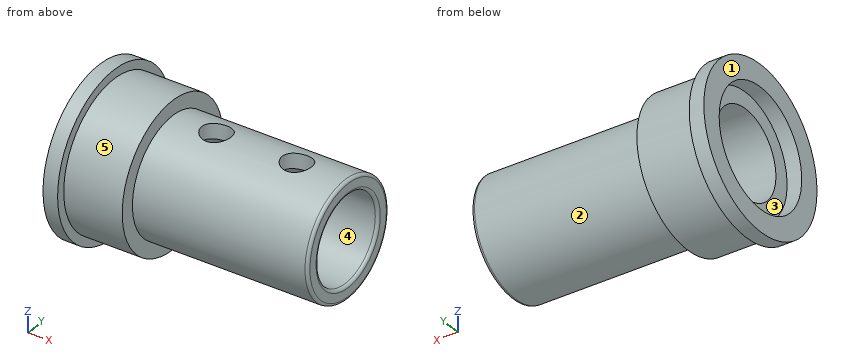
```python
from build123d import *

# Parameters (mm, degrees)
ESQUISSE4_W               = 1
ESQUISSE4_H               = 5.55
D_GAGEMENT_M21_AT_2_COUNT = 2
D_GAGEMENT_M21_AT_2_PITCH = 5.5


with BuildPart() as part:
    # Esquisse1 → Révolution1 (revolve)
    with BuildSketch(Plane.XY):
        with BuildLine():
            Line((0, 4.05), (0, 5.55))
            Line((0, 5.55), (1, 5.55))
            Line((1, 5.55), (1, 4.95))
            Line((1, 4.95), (5, 4.95))
            Line((5, 4.95), (5, 3.95))
            Line((5, 3.95), (16.8, 3.95))
            ThreePointArc((16.8, 3.95), (16.941421356, 3.891421356), (17, 3.75))
            Line((17, 3.75), (17, 3.15))
            ThreePointArc((17, 3.15), (16.941421356, 3.008578644), (16.8, 2.95))
            Line((16.8, 2.95), (1, 2.95))
            Line((1, 2.95), (1, 4.05))
            Line((1, 4.05), (0, 4.05))
        make_face()
    revolve(axis=Axis((-11.300588411, 0, 0), (1, 0, 0)))

    # Esquisse4 → Dégagement M21 (revolve, cut)
    with BuildSketch(Plane.YZ.offset(8)):
        with Locations((0.5, 2.775)):
            Rectangle(ESQUISSE4_W, ESQUISSE4_H)
    d_gagement_m21 = revolve(axis=Axis((8, 0, -6.35), (0, 0, 1)), mode=Mode.SUBTRACT)

    # Dégagement M21 at 2: Dégagement M21 ×2
    with Locations(*[(i * D_GAGEMENT_M21_AT_2_PITCH, 0, 0) for i in range(1, D_GAGEMENT_M21_AT_2_COUNT)]):
        add(d_gagement_m21, mode=Mode.SUBTRACT)


solid = part.part
```
Read the model definition and answer for the solid it produces. Units are mm, in the model's axes. Face numbers are marked on the shaded views. A direction names the side the tool comes from. Give positions to 0.01 mm unless a question says otherwise; leave off trailing zeros. Order: outer loops, then holes, each group sorted by start corner. A loop starts at its lowest first (then second) coordinate and runs counter-clockwise, first axis right, second up.
(1) Find section D-D (y = -4.5). Give the vertices of the cut face in (x, z), plus the area to 3 significant figures.
(2) Find section B-B (y = 0). Give the number of separate pieces and of enclosed holes in the cut face, plus the area to 3 significant figures.
(3) For the marked faces 4 and 5, determine the directions among +Z, -Z, +X, -X, +Y, -Y from which every point of the face is accessible in a straight line to the end or side of a thin tool.
(4) Straight lines are drawn through the part: L1, parallel to X at y = 0, z = 3.6; L2, parallel to Z at x = 11.75, y = 0; L3, parallel to Z at x = 0.6, y = 0. For each, find the intervals that lie inside material, in ascending order.
(5) Find section C-C (x = 1.75). Give the vertices of the cut face in (y, z).
(6) For a pull along Y with two mould halves and no side action, classify the marked faces 1, 2 and 3 as released by +Y, released by -Y, zero draft, split by the parting line, or undercut.
(7) Given pin 1 (3 mm diameter, centred on x = 8, y = 0, fed in from -Z); pin 2 (2 mm diameter, centred on x = 9.5, z = 3.5, fed in from -Y); pin 3 (1.5 mm diameter, centred on x = 8.5, z = 3, fed in from +Y), each flat-ended and moving along its own axis, determine where each tip first touches the part or whether it passes through.
(8) Find section A-A (z = 0). Give the vertices of the cut face in (x, y).
Result sheet:
1. outline: (0, -3.25) - (1, -3.25) - (1, -2.06) - (5, -2.06) - (5, 2.06) - (1, 2.06) - (1, 3.25) - (0, 3.25) - close
1. area: 23.0 mm2
2. separate pieces: 4
2. enclosed holes: 0
2. area: 39.0 mm2
3. face 4: +X, -X
3. face 5: +X
4. L1: x = 1 to 7, 9 to 12.5, 14.5 to 17
4. L2: z = -3.95 to -2.95, 2.95 to 3.95
4. L3: z = -5.55 to -4.05, 4.05 to 5.55
5. outline: circle Ø9.9 at (0, 0); hole circle Ø5.9 at (0, 0)
6. face 1: zero draft
6. face 2: split by the parting line
6. face 3: undercut
7. pin 1: stops at z = -3.95
7. pin 2: stops at y = -3.06
7. pin 3: stops at y = 3.25
8. outline: (0, -5.55) - (1, -5.55) - (1, -4.95) - (5, -4.95) - (5, -3.95) - (16.8, -3.95) arc R0.2 ccw to (17, -3.75) - (17, -3.15) arc R0.2 ccw to (16.8, -2.95) - (1, -2.95) - (1, -4.05) - (0, -4.05) - close; (0, 4.05) - (1, 4.05) - (1, 2.95) - (16.8, 2.95) arc R0.2 ccw to (17, 3.15) - (17, 3.75) arc R0.2 ccw to (16.8, 3.95) - (5, 3.95) - (5, 4.95) - (1, 4.95) - (1, 5.55) - (0, 5.55) - close
